from build123d import *

# Parameters (mm, degrees)
F1_DEPTH = 1.5
F2_DEPTH = 10
F3_SIZE  = 1


with BuildPart() as f1:
    # F0 (on Top) → F1 (new body)
    with BuildSketch(Plane.XY):
        with BuildLine():
            ThreePointArc((102.5, 60), (101.035534, 63.535534), (97.5, 65))
            Line((97.5, 65), (-97.5, 65))
            ThreePointArc((-97.5, 65), (-101.035534, 63.535534), (-102.5, 60))
            Line((-102.5, 60), (-102.5, -60))
            ThreePointArc((-102.5, -60), (-101.035534, -63.535534), (-97.5, -65))
            Line((-97.5, -65), (97.5, -65))
            ThreePointArc((97.5, -65), (101.035534, -63.535534), (102.5, -60))
            Line((102.5, -60), (102.5, 60))
        make_face()
    extrude(amount=F1_DEPTH)

    # F0 (on Top) → F2 (join)
    with BuildSketch(Plane.XY):
        with BuildLine():
            Line((104.3, -60), (104.3, 60))
            ThreePointArc((104.3, 60), (102.308326, 64.808326), (97.5, 66.8))
            Line((97.5, 66.8), (-97.5, 66.8))
            ThreePointArc((-97.5, 66.8), (-102.308326, 64.808326), (-104.3, 60))
            Line((-104.3, 60), (-104.3, -60))
            ThreePointArc((-104.3, -60), (-102.308326, -64.808326), (-97.5, -66.8))
            Line((-97.5, -66.8), (97.5, -66.8))
            ThreePointArc((97.5, -66.8), (102.308326, -64.808326), (104.3, -60))
        make_face()
        with BuildLine():
            Line((-97.5, 65), (97.5, 65))
            ThreePointArc((97.5, 65), (101.035534, 63.535534), (102.5, 60))
            Line((102.5, 60), (102.5, -60))
            ThreePointArc((102.5, -60), (101.035534, -63.535534), (97.5, -65))
            Line((97.5, -65), (-97.5, -65))
            ThreePointArc((-97.5, -65), (-101.035534, -63.535534), (-102.5, -60))
            Line((-102.5, -60), (-102.5, 60))
            ThreePointArc((-102.5, 60), (-101.035534, 63.535534), (-97.5, 65))
        make_face(mode=Mode.SUBTRACT)
    extrude(amount=F2_DEPTH)

    # F3
    f3_edges = [f1.edges().sort_by_distance(p)[0] for p in [
        (102.308326, -64.808326, 0),
        (104.3, 0, 0),
        (102.308326, 64.808326, 0),
        (0, 66.8, 0),
        (-102.308326, 64.808326, 0),
        (-104.3, 0, 0),
        (-102.308326, -64.808326, 0),
        (0, -66.8, 0),
        (101.035534, 63.535534, 1.5),
        (0, 65, 1.5),
        (-101.035534, 63.535534, 1.5),
        (-102.5, 0, 1.5),
        (-101.035534, -63.535534, 1.5),
        (0, -65, 1.5),
        (101.035534, -63.535534, 1.5),
        (102.5, 0, 1.5),
        (97.5, 65, 5.75),
        (0, 65, 10),
        (-97.5, 65, 5.75),
    ]]
    chamfer(f3_edges, length=F3_SIZE)


solid = f1.part
Work out the finished part from the listing and answer in its coordinate system (mm). A direction names the side the tool comes from. Coordinates: 2 decimals unless noted, no trailing zeros. Write each loop counter-clockwise with the first axis right and the second up, starting at its lowest first coordinate (ties: lowest second). Pieces come first, ordered by that corner, then holes.
1. The part is cut by section C-C, the plane x = -58. Write down the section's boundary in (y, z), and give its area (3 significant figures).
Results list:
outline: (-66.8, 1) - (-65.8, 0) - (65.8, 0) - (66.8, 1) - (66.8, 10) - (66, 10) - (65, 9) - (65, 2.5) - (64, 1.5) - (-64, 1.5) - (-65, 2.5) - (-65, 9) - (-66, 10) - (-66.8, 10) - close
area: 230 mm2
2. For faces 5 (the conical face through (-101.67, 64.26, 0.16)), 6 (the flat face through (-1, 1, 1.5)), determine the directions among +Z, -Z, +X, -X, +Y, -Y from which every point of the face is accessible in a straight line to the end or side of a thin tool.
Results list:
face 5: -Z, -X, +Y
face 6: +Z
3. Consider line 1 along Y through (x, z) = (-40, 7.75); line 2 along X through (y, z) = (35, 4); line 3 along Z through (x, y) = (46, -12). Determine where each line is inside the solid, lowest interval first.
Results list:
line 1: y = -66.8 to -65, 65 to 66.8
line 2: x = -104.3 to -102.5, 102.5 to 104.3
line 3: z = 0 to 1.5
4. The part is cut by section B-B, the plane y = -40. Write down the section's boundary in (x, z), and give its area (4 significant figures).
Results list:
outline: (-104.3, 1) - (-103.3, 0) - (103.3, 0) - (104.3, 1) - (104.3, 10) - (103.5, 10) - (102.5, 9) - (102.5, 2.5) - (101.5, 1.5) - (-101.5, 1.5) - (-102.5, 2.5) - (-102.5, 9) - (-103.5, 10) - (-104.3, 10) - close
area: 342.5 mm2
5. For a pull along Y with two mould halves and no side action, classify faces 1 (the cylindrical face through (102.255, -64.861, 5.437)), 2 (the flat face through (-1, 1, 0)), 3 (the conical face through (101.186, 63.768, 9.271)), 4 (the cylindrical face through (-101, -63.57, 5.7)) as +Y half, -Y half, draft (parallel to the pull), parting line (faces both ways), or undercut.
Results list:
face 1: -Y half
face 2: draft
face 3: undercut
face 4: undercut
6. A flat-ended cylindrical pin translates along its axis: pin 1 (6 mm diameter, centred on x = -36.5, y = -9, fed in from +Z). Find the tip coordinate at first contact, or state that the pin passes through.
Results list:
pin 1: stops at z = 1.5
7. The part is cut by section A-A, the plane z = 6.75. Write down the section's boundary in (x, y).
Results list:
outline: (-104.3, -60) arc R6.8 ccw to (-97.5, -66.8) - (97.5, -66.8) arc R6.8 ccw to (104.3, -60) - (104.3, 60) arc R6.8 ccw to (97.5, 66.8) - (-97.5, 66.8) arc R6.8 ccw to (-104.3, 60) - close; hole (-102.5, -60) arc R5 ccw to (-97.5, -65) - (97.5, -65) arc R5 ccw to (102.5, -60) - (102.5, 60) arc R5 ccw to (97.5, 65) - (-97.5, 65) arc R5 ccw to (-102.5, 60) - close
